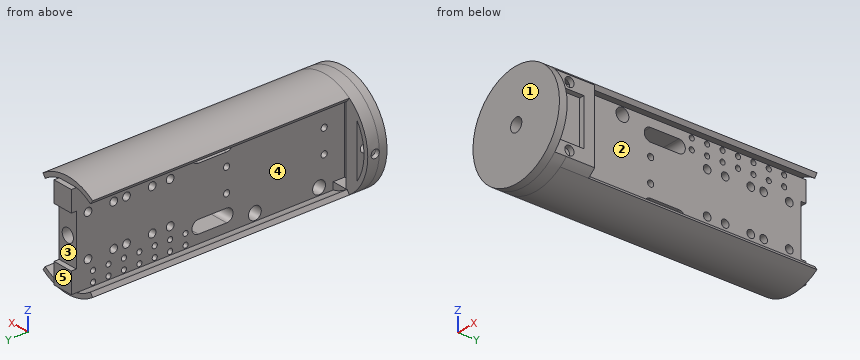
from build123d import *
from build123d.topology import SkipClean

# Parameters (mm, degrees)
SKETCH1_R            = 25.4
SKETCH1_R_2          = 3.302
BOTTOM_PLATE_DEPTH   = 3.81
LIP_START            = 5.715
SKETCH1_4_R          = 3.302
LIP_DEPTH            = 5.715
BOSS_EXTRUDE1_START  = 127
SKETCH2_R            = 3.302
BOSS_EXTRUDE1_DEPTH  = 127
SKETCH3_R            = 3.175
SKETCH3_R_2          = 1.524
SKETCH3_R_3          = 1.905
SKETCH3_R_4          = 1.27
MOUNTING_HOLES_DEPTH = 10.16
SKETCH4_W            = 10.16
SKETCH4_H            = 10.16
NOTCHES_DEPTH        = 2.54
SWITCH_FACE_START    = 13.97
SWITCH_FACE_DEPTH    = 13.97
SKETCH8_R            = 2.286
SKETCH8_W            = 22.86
SKETCH8_H            = 14.478
SWITCH_MOUNT_DEPTH   = 6.35
INDICATOR_CUT_START  = -43.539228
SKETCH8_3_R          = 2.032
INDICATOR_CUT_DEPTH  = 12.7


with BuildPart() as part:
    # Sketch1 → bottom_plate (new body)
    with BuildSketch(Plane(origin=(0, 0, 0), x_dir=(1, 0, 0), z_dir=(0, 1, 0))):
        with Locations(Location((0, 0, 0), (0, 0, 270))):
            Circle(SKETCH1_R)
        with Locations(Location((0, 0, 0), (0, 0, 270))):
            Circle(SKETCH1_R_2, mode=Mode.SUBTRACT)
    extrude(amount=-BOTTOM_PLATE_DEPTH)

    # Sketch1<4> → lip (add)
    # profile 1 of 3: a face of its own
    with BuildSketch(Plane(origin=(0, 0, 0), x_dir=(1, 0, 0), z_dir=(0, 1, 0)).offset(LIP_START)):
        with BuildLine():
            Line((18.139228208, -17.78), (18.139228208, 17.78))
            ThreePointArc((18.139228208, 17.78), (-25.4, 0), (18.139228208, -17.78))
        make_face()
        with BuildLine():
            ThreePointArc((15.599228208, -17.142362309), (-23.1775, 0), (15.599228208, 17.142362309))
            Line((15.599228208, 17.142362309), (15.599228208, -17.142362309))
        make_face(mode=Mode.SUBTRACT)
    # profile 2 of 3: a face of its own
    with BuildSketch(Plane(origin=(0, 0, 0), x_dir=(1, 0, 0), z_dir=(0, 1, 0)).offset(LIP_START)):
        with BuildLine():
            ThreePointArc((5.08, 22.613936107), (0, 23.1775), (-5.08, 22.613936107))
            Line((-5.08, 22.613936107), (-5.08, 19.05))
            Line((-5.08, 19.05), (-5.08, -19.05))
            Line((-5.08, -19.05), (-5.08, -22.613936107))
            ThreePointArc((-5.08, -22.613936107), (0, -23.1775), (5.08, -22.613936107))
            Line((5.08, -22.613936107), (5.08, 22.613936107))
        make_face()
        with Locations(Location((0, 0, 0), (0, 0, 270))):
            Circle(SKETCH1_4_R, mode=Mode.SUBTRACT)
    # profile 3 of 3: a face of its own
    with BuildSketch(Plane(origin=(0, 0, 0), x_dir=(1, 0, 0), z_dir=(0, 1, 0)).offset(LIP_START)):
        with BuildLine():
            Line((-5.08, 19.05), (-5.08, 22.613936107))
            ThreePointArc((-5.08, 22.613936107), (-12.950295211, 19.222027994), (-19.05, 13.202045533))
            Line((-19.05, 13.202045533), (-19.05, -13.202045533))
            ThreePointArc((-19.05, -13.202045533), (-12.950295211, -19.222027994), (-5.08, -22.613936107))
            Line((-5.08, -22.613936107), (-5.08, -19.05))
            Line((-5.08, -19.05), (-12.7, -19.05))
            Line((-12.7, -19.05), (-12.7, 19.05))
            Line((-12.7, 19.05), (-5.08, 19.05))
        make_face()
    extrude(amount=-LIP_DEPTH)

    # Sketch2 → Boss-Extrude1 (add)
    with SkipClean():  # the faces are left unmerged after this step: merging them gives an invalid solid
        with BuildSketch(Plane(origin=(0, 5.715, 0), x_dir=(1, 0, 0), z_dir=(0, 1, 0)).offset(BOSS_EXTRUDE1_START)):
            with BuildLine():
                Line((5.08, 22.613936107), (5.08, -22.613936107))
                ThreePointArc((5.08, -22.613936107), (9.364414568, -21.201515183), (13.294067854, -18.985896507))
                Line((13.294067854, -18.985896507), (14.568841483, -20.806461925))
                ThreePointArc((14.568841483, -20.806461925), (0, -25.4), (-14.568841483, -20.806461925))
                Line((-14.568841483, -20.806461925), (-13.294067854, -18.985896507))
                ThreePointArc((-13.294067854, -18.985896507), (-9.364414568, -21.201515183), (-5.08, -22.613936107))
                Line((-5.08, -22.613936107), (-5.08, 22.613936107))
                ThreePointArc((-5.08, 22.613936107), (-9.364414568, 21.201515183), (-13.294067854, 18.985896507))
                Line((-13.294067854, 18.985896507), (-14.568841483, 20.806461925))
                ThreePointArc((-14.568841483, 20.806461925), (0, 25.4), (14.568841483, 20.806461925))
                Line((14.568841483, 20.806461925), (13.294067854, 18.985896507))
                ThreePointArc((13.294067854, 18.985896507), (9.364414568, 21.201515183), (5.08, 22.613936107))
            make_face()
            with Locations(Location((0, 0, 0), (0, 0, 270))):
                Circle(SKETCH2_R, mode=Mode.SUBTRACT)
        extrude(amount=-BOSS_EXTRUDE1_DEPTH)

    # Sketch3 → mounting_holes (cut)
    with SkipClean():  # the faces are left unmerged after this step: merging them gives an invalid solid
        with BuildSketch(Plane.ZY.offset(5.08)):
            with BuildLine():
                Line((18.415, 58.42), (18.415, 72.39))
                ThreePointArc((18.415, 72.39), (15.24, 75.565), (12.065, 72.39))
                Line((12.065, 72.39), (12.065, 58.42))
                ThreePointArc((12.065, 58.42), (15.24, 55.245), (18.415, 58.42))
            make_face()
            with BuildLine():
                Line((-12.065, 58.42), (-12.065, 72.39))
                ThreePointArc((-12.065, 72.39), (-15.24, 75.565), (-18.415, 72.39))
                Line((-18.415, 72.39), (-18.415, 58.42))
                ThreePointArc((-18.415, 58.42), (-15.24, 55.245), (-12.065, 58.42))
            make_face()
            with Locations((-19.05, 44.45)):
                Circle(SKETCH3_R)
            with Locations((19.05, 44.45)):
                Circle(SKETCH3_R)
            with Locations((-19.05, 12.7)):
                Circle(SKETCH3_R)
            with Locations((19.05, 12.7)):
                Circle(SKETCH3_R)
            with Locations((-5.715, 58.42)):
                Circle(SKETCH3_R_2)
            with Locations((5.715, 58.42)):
                Circle(SKETCH3_R_2)
            with Locations((-5.715, 10.16)):
                Circle(SKETCH3_R_2)
            with Locations((5.715, 10.16)):
                Circle(SKETCH3_R_2)
            with Locations((10.16, 86.36)):
                Circle(SKETCH3_R_3)
            with Locations((-10.16, 86.36)):
                Circle(SKETCH3_R_3)
            with Locations((-10.16, 107.95)):
                Circle(SKETCH3_R_3)
            with Locations((-10.16, 95.25)):
                Circle(SKETCH3_R_3)
            with Locations((10.16, 107.95)):
                Circle(SKETCH3_R_3)
            with Locations((10.16, 95.25)):
                Circle(SKETCH3_R_3)
            with Locations((-10.16, 127)):
                Circle(SKETCH3_R_3)
            with Locations((-10.16, 114.3)):
                Circle(SKETCH3_R_3)
            with Locations((10.16, 114.3)):
                Circle(SKETCH3_R_3)
            with Locations((10.16, 127)):
                Circle(SKETCH3_R_3)
            with Locations((-20.955, 78.74)):
                Circle(SKETCH3_R_4)
            with Locations((-15.875, 78.74)):
                Circle(SKETCH3_R_4)
            with Locations((-20.955, 86.36)):
                Circle(SKETCH3_R_4)
            with Locations((-15.875, 86.36)):
                Circle(SKETCH3_R_4)
            with Locations((-20.955, 93.98)):
                Circle(SKETCH3_R_4)
            with Locations((-15.875, 93.98)):
                Circle(SKETCH3_R_4)
            with Locations((-20.955, 101.6)):
                Circle(SKETCH3_R_4)
            with Locations((-15.875, 101.6)):
                Circle(SKETCH3_R_4)
            with Locations((-20.955, 109.22)):
                Circle(SKETCH3_R_4)
            with Locations((-15.875, 109.22)):
                Circle(SKETCH3_R_4)
            with Locations((-20.955, 116.84)):
                Circle(SKETCH3_R_4)
            with Locations((-15.875, 116.84)):
                Circle(SKETCH3_R_4)
            with Locations((-20.955, 124.46)):
                Circle(SKETCH3_R_4)
            with Locations((-15.875, 124.46)):
                Circle(SKETCH3_R_4)
            with Locations((20.955, 124.46)):
                Circle(SKETCH3_R_4)
            with Locations((15.875, 124.46)):
                Circle(SKETCH3_R_4)
            with Locations((15.875, 116.84)):
                Circle(SKETCH3_R_4)
            with Locations((20.955, 116.84)):
                Circle(SKETCH3_R_4)
            with Locations((20.955, 109.22)):
                Circle(SKETCH3_R_4)
            with Locations((15.875, 109.22)):
                Circle(SKETCH3_R_4)
            with Locations((15.875, 101.6)):
                Circle(SKETCH3_R_4)
            with Locations((20.955, 101.6)):
                Circle(SKETCH3_R_4)
            with Locations((20.955, 93.98)):
                Circle(SKETCH3_R_4)
            with Locations((15.875, 93.98)):
                Circle(SKETCH3_R_4)
            with Locations((20.955, 86.36)):
                Circle(SKETCH3_R_4)
            with Locations((15.875, 86.36)):
                Circle(SKETCH3_R_4)
            with Locations((20.955, 78.74)):
                Circle(SKETCH3_R_4)
            with Locations((15.875, 78.74)):
                Circle(SKETCH3_R_4)
        extrude(amount=-MOUNTING_HOLES_DEPTH, mode=Mode.SUBTRACT)

    # Sketch4 → notches (add)
    with SkipClean():  # the faces are left unmerged after this step: merging them gives an invalid solid
        with BuildSketch(Plane(origin=(0, 132.715, 0), x_dir=(1, 0, 0), z_dir=(0, 1, 0))):
            with Locations((0, 17.533936107)):
                Rectangle(SKETCH4_W, SKETCH4_H)
            with Locations((0, -17.533936107)):
                Rectangle(SKETCH4_W, SKETCH4_H)
        extrude(amount=NOTCHES_DEPTH)

    # Sketch7 → switch_face (add)
    with SkipClean():  # the faces are left unmerged after this step: merging them gives an invalid solid
        with BuildSketch(Plane(origin=(0, 5.715, 0), x_dir=(1, 0, 0), z_dir=(0, 1, 0)).offset(SWITCH_FACE_START)):
            with BuildLine():
                Line((13.294067854, -18.985896507), (14.568841483, -20.806461925))
                ThreePointArc((14.568841483, -20.806461925), (16.4238949, -19.375646475), (18.139228208, -17.78))
                Line((18.139228208, -17.78), (18.139228208, 17.78))
                ThreePointArc((18.139228208, 17.78), (16.4238949, 19.375646475), (14.568841483, 20.806461925))
                Line((14.568841483, 20.806461925), (13.294067854, 18.985896507))
                ThreePointArc((13.294067854, 18.985896507), (14.476024797, 18.100862199), (15.599228208, 17.142362309))
                Line((15.599228208, 17.142362309), (15.599228208, -17.142362309))
                ThreePointArc((15.599228208, -17.142362309), (14.476024797, -18.100862199), (13.294067854, -18.985896507))
            make_face()
        extrude(amount=-SWITCH_FACE_DEPTH)

    # Sketch8 → switch_mount (cut)
    with SkipClean():  # the faces are left unmerged after this step: merging them gives an invalid solid
        with BuildSketch(Plane(origin=(18.139228208, 0, 0), x_dir=(0, 0, -1), z_dir=(1, 0, 0))):
            with Locations((14.732, 7.239)):
                Circle(SKETCH8_R)
            with Locations((-14.732, 7.239)):
                Circle(SKETCH8_R)
            with Locations((0, 7.239)):
                Rectangle(SKETCH8_W, SKETCH8_H)
        extrude(amount=-SWITCH_MOUNT_DEPTH, mode=Mode.SUBTRACT)

    # Sketch8<3> → indicator_cut (cut)
    with SkipClean():  # the faces are left unmerged after this step: merging them gives an invalid solid
        with BuildSketch(Plane(origin=(18.139228208, 0, 0), x_dir=(0, 0, -1), z_dir=(1, 0, 0)).offset(INDICATOR_CUT_START)):
            with Locations(Location((0, 2.032, 0), (0, 0, 270))):
                Circle(SKETCH8_3_R)
        extrude(amount=INDICATOR_CUT_DEPTH, mode=Mode.SUBTRACT)


solid = part.part
Input: part model. Units: mm. Frame: model coordinates. Face numbers are marked on the shaded views. A direction names the side the tool comes from. Round coordinates to 2 decimals unless told otherwise and drop trailing zeros. Order: outer loops, then holes, each group sorted by start corner. A loop starts at its lowest first (then second) coordinate and runs counter-clockwise, first axis right, second up.
1. Mould query, pull axis X, two halves, no side actions, for the marked faces 4 and 5. Classes: released by +X, released by -X, zero draft, split by the parting line, or undercut.
The answers:
face 4: undercut
face 5: zero draft
2. Cut plane A-A, the plane y = 78.74. State how many separate pieces and enclosed holes the cut face has, then the cut area to 3 significant figures.
The answers:
separate pieces: 5
enclosed holes: 1
area: 462 mm2
3. Pin query (flat end, axial travel): P1, Ø3.5, axis at y = 93.98, z = -20.955, coming from the +X side; P2, Ø1.3, axis at x = -2, y = 134.5, coming from the -Z side; P3, Ø7.5, axis at y = 7.239, z = 14.732, coming from the -X side; P4, Ø6.5, axis at y = 2.032, z = 0, coming from the +X side. Return the tip coordinate at first contact, or that it passes through.
The answers:
P1: stops at x = 14.57
P2: stops at z = -22.61
P3: stops at x = -22.75
P4: stops at x = 25.4
4. Set-up query: the marked faces 1, 2 and 3. Return all of +Z, -Z, +X, -X, +Y, -Y with unobstructed straight access to the full face (end or side cutting, diameter ignored); none if empty.
The answers:
face 1: +Z, -Z, +X, -X, -Y
face 2: +Y
face 3: +X, -X, +Y
5. Material intervals for line 1 (Y direction, x = 2.75, z = -10.16) (3 decimals); line 2 (X direction, y = 107, z = 0); line 3 (Y direction, x = -5, z = 18) (3 decimals), sorted ascending.
The answers:
line 1: y = -3.81 to 84.455, 88.265 to 93.345, 97.155 to 106.045, 109.855 to 112.395, 116.205 to 125.095, 128.905 to 132.715
line 2: x = -5.08 to -3.3, 3.3 to 5.08
line 3: y = -3.81 to 9.704, 15.696 to 41.454, 47.446 to 56.851, 73.959 to 135.255
6. Cut plane D-D, the plane x = -17. Output: boundary loops of the cut face in (y, z) (3 decimals), then the cut area to 3 significant figures.
The answers:
outline: (-3.81, -18.872) - (5.715, -18.872) - (5.715, 18.872) - (-3.81, 18.872) - close; hole circle Ø4.064 at (2.032, 0)
area: 347 mm2
7. Cut plane B-B, the plane y = 49.5. Output: boundary loops of the cut face in (x, z) (1 decimal), then the cut area to 3 significant figures.
The answers:
outline: (-14.6, -20.8) arc R25.4 ccw to (14.6, -20.8) - (13.3, -19) arc R23.2 cw to (5.1, -22.6) - (5.1, 22.6) arc R23.2 cw to (13.3, 19) - (14.6, 20.8) arc R25.4 ccw to (-14.6, 20.8) - (-13.3, 19) arc R23.2 cw to (-5.1, 22.6) - (-5.1, -22.6) arc R23.2 cw to (-13.3, -19) - close; hole circle Ø6.6 at (0, 0)
area: 565 mm2
